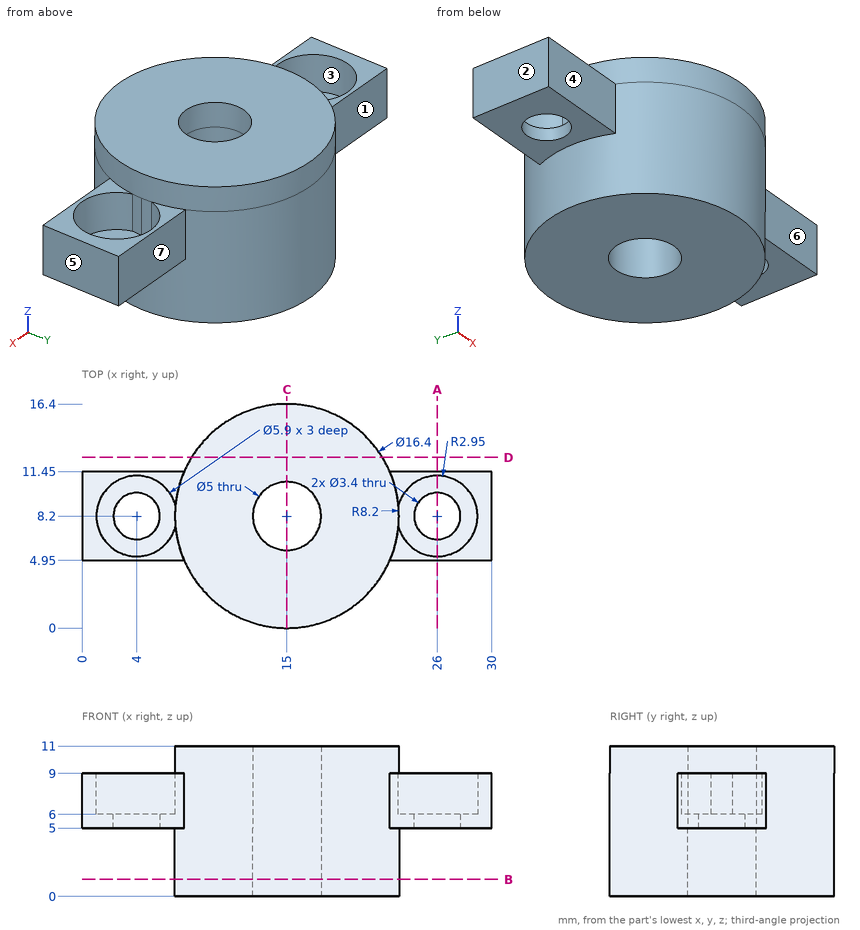
The drawing under review shows one solid part. Ordinate dimensions are in mm from its lowest x, y, z. A direction names the side the tool comes from. Coordinates: 2 decimals unless noted, no trailing zeros. Loops run counter-clockwise (first coordinate to the right, second up) from the corner with the lowest first, then second, coordinate; pieces in that order, holes last.
Item 1: Add section C-C (x = 15). Write out the cut boundary in (y, z).
Completed:
outline: (0, 0) - (5.7, 0) - (5.7, 11) - (0, 11) - close; (10.7, 0) - (16.4, 0) - (16.4, 11) - (10.7, 11) - close
Item 2: Add section A-A (x = 26). Write out the cut boundary in (y, z).
Completed:
outline: (4.95, 5) - (6.5, 5) - (6.5, 6) - (5.25, 6) - (5.25, 9) - (4.95, 9) - close; (9.9, 5) - (11.45, 5) - (11.45, 9) - (11.15, 9) - (11.15, 6) - (9.9, 6) - close
Item 3: Add section B-B (z = 1.25). Write out the cut boundary in (x, y), and give its area (3 significant figures).
Completed:
outline: circle Ø16.4 at (15, 8.2); hole circle Ø5 at (15, 8.2)
area: 192 mm2
Item 4: Draft analysis for pull direction X (two halves, no side actions). For the marked faces 1, 2 and 3, state which applies: pulls with the +X half, pulls with the -X half, needs draft (parallel to the pull), parting line crosses it, or undercut.
Completed:
face 1: needs draft
face 2: pulls with the -X half
face 3: undercut
Item 5: For the marked faces 4, 5, 6 and 7, list the 3-axis set-ups (+Z, -Z, +X, -X, +Y, -Y) from which the entire face can be reached by the end or side of a thin tool; tool diameter is ignored.
Completed:
face 4: +Z, -Z, -X, -Y
face 5: +Z, -Z, +X, +Y, -Y
face 6: +Z, -Z, +X, -Y
face 7: +Z, -Z, +X, +Y
Item 6: Add section D-D (y = 12.5). Write out the cut boundary in (x, z), and give its area (3 significant figures).
Completed:
outline: (8.02, 0) - (21.98, 0) - (21.98, 11) - (8.02, 11) - close
area: 154 mm2
Item 7: Wall thickness on L1, parallel to Y at x = 15, z = 7.2; L2, parallel to X at y = 10, z = 10.75; L3, parallel to Y at x = 16, z = 8: over which ranges is each line inside the solid? List them lowest first.
Completed:
L1: y = 0 to 5.7, 10.7 to 16.4
L2: x = 7 to 13.27, 16.73 to 23
L3: y = 0.06 to 5.91, 10.49 to 16.34
Item 8: Clearance check with flat-ended pins moving along their axes: pin 1 (3 mm diameter, centred on x = 27.5, z = 7, fed in from -Y); pin 2 (5.5 mm diameter, centred on x = 26, y = 8.2, fed in from -Z); pin 3 (1 mm diameter, centred on y = 2.5, z = 9, fed in from -X). State where each tip first meets the part, or that it passes through.
Completed:
pin 1: stops at y = 4.95
pin 2: stops at z = 5
pin 3: stops at x = 8.66
